The model under review builds one solid part; all positions refer to its coordinate system, in mm. A direction names the side the tool comes from. Round coordinates to 2 decimals unless told otherwise and drop trailing zeros. Loops run counter-clockwise (first coordinate to the right, second up) from the corner with the lowest first, then second, coordinate; pieces in that order, holes last. Notation, with made-up numbers: (29, 67) -> (52, 67) arc R20 cw to (52, 105) -> close; hole circle Ø10 at (62, 47). An arc over 180 degrees is marked (long way). Return JSON: item names as keys, results as strings. Group by question number.
```python
from build123d import *

# Parameters (mm, degrees)
BOSS_EXTRUDE1_DEPTH = 4
CUT_EXTRUDE1_DEPTH  = 5
CUT_EXTRUDE3_DEPTH  = 5
CUT_EXTRUDE4_DEPTH  = 5
CUT_EXTRUDE5_DEPTH  = 5
SHELL1_T            = -1.5


with BuildPart() as part:
    # Sketch1 → Boss-Extrude1 (new body)
    with BuildSketch(Plane(origin=(0, 0, 0), x_dir=(1, 0, 0), z_dir=(0, 1, 0))):
        Polygon((-87.851196474, 52.910261526), (152.148803526, 52.910261526), (182.148803526, 22.910261526), (182.148803526, -167.089738474), (152.148803526, -197.089738474), (-87.851196474, -197.089738474), (-117.851196474, -167.089738474), (-117.851196474, 22.910261526), align=None)
    extrude(amount=BOSS_EXTRUDE1_DEPTH)

    # Sketch2 → Cut-Extrude1 (cut)
    with BuildSketch(Plane(origin=(0, 4, 0), x_dir=(1, 0, 0), z_dir=(0, 1, 0))):
        Polygon((-75.981138789, -72.089738474), (-75.981138789, -32.089738474), (-117.851196474, 9.780319211), (-117.851196474, -153.959796159), (-75.981138789, -112.089738474), align=None)
    extrude(amount=-CUT_EXTRUDE1_DEPTH, mode=Mode.SUBTRACT)

    # Sketch2_5 → Cut-Extrude3 (cut)
    with BuildSketch(Plane(origin=(0, 4, 0), x_dir=(1, 0, 0), z_dir=(0, 1, 0))):
        Polygon((140.278745841, -72.089738474), (140.278745841, -112.089738474), (182.148803526, -153.959796159), (182.148803526, 9.780319211), (140.278745841, -32.089738474), align=None)
    extrude(amount=-CUT_EXTRUDE3_DEPTH, mode=Mode.SUBTRACT)

    # Sketch2_6 → Cut-Extrude4 (cut)
    with BuildSketch(Plane(origin=(0, 4, 0), x_dir=(1, 0, 0), z_dir=(0, 1, 0))):
        Polygon((-61.839003165, 11.040203841), (-90.123274413, 39.324475088), (-104.265410036, 25.182339465), (-75.981138789, -3.101931783), (-68.910070977, 3.969136029), align=None)
        Polygon((126.136610217, 11.040203841), (154.420881465, 39.324475088), (168.563017088, 25.182339465), (140.278745841, -3.101931783), (133.207678029, 3.969136029), align=None)
        Polygon((168.563017088, -169.361816413), (154.420881465, -183.503952036), (126.136610217, -155.219680789), (133.207678029, -148.148612977), (140.278745841, -141.077545165), align=None)
        Polygon((-104.702510795, -169.798917171), (-90.550656516, -183.95077145), (-61.839003165, -155.219680789), (-68.910070977, -148.148612977), (-75.981138789, -141.077545165), align=None)
    extrude(amount=-CUT_EXTRUDE4_DEPTH, mode=Mode.SUBTRACT)

    # Sketch2_7 → Cut-Extrude5 (cut)
    with BuildSketch(Plane(origin=(0, 4, 0), x_dir=(1, 0, 0), z_dir=(0, 1, 0))):
        Polygon((139.018803526, 52.910261526), (32.148803526, 52.910261526), (32.148803526, 11.040203841), (97.148861211, 11.040203841), align=None)
        Polygon((32.148803526, 11.040203841), (32.148803526, 52.910261526), (-74.721196474, 52.910261526), (-32.851138789, 11.040203841), align=None)
        Polygon((-74.721196474, -197.089738474), (32.148803526, -197.089738474), (32.148803526, -155.219680789), (-32.851138789, -155.219680789), align=None)
        Polygon((32.148803526, -155.219680789), (32.148803526, -197.089738474), (139.018803526, -197.089738474), (97.148861211, -155.219680789), align=None)
    extrude(amount=-CUT_EXTRUDE5_DEPTH, mode=Mode.SUBTRACT)

    # Shell1
    shell1_openings = [part.faces().sort_by_distance(p)[0] for p in [
        (147.349813653, 4, 162.290748601),
    ]]
    offset(amount=SHELL1_T, openings=shell1_openings, kind=Kind.INTERSECTION)


solid = part.part
```
1. Wall thickness on line 1 (Z direction, x = -0.5, y = 2.65); line 2 (X direction, y = 0.9, z = -13.5); line 3 (X direction, y = 3.5, z = -2): over which ranges is each line inside the solid? List them lowest first.
2. We need section D-D, the plane x = 18.5. Write out the cut boundary in (y, z).
3. For P1, Ø2, axis at y = 1, z = 80.5, coming from the +X side; P2, Ø1, axis at y = 2.5, z = 115.5, coming from the -X side; P3, Ø1.5, axis at x = -59, z = 141.5, coming from the +Y side, all flat-tipped, find the tip position at first contact; note any pin that passes through.
4. Tool access review of faces 1 (the face through (133.109, 2.028, -4.068)), 2 (the face through (154, 4, -10)), 3 (the face through (-95.12, 2.77, 10.83)): name each direction out of +Z, -Z, +X, -X, +Y, -Y from which nothing blocks a thin tool from reaching the whole face with its end or side.
5. We need section B-B, the plane z = 49. Write out the cut boundary in (x, y), then the cut area to 3 significant figures.
6. We need section C-C, the plane y = 3.05. Give the number of separate pieces and of enclosed holes in the cut face, then the cut area to 3 significant figures.
7. We need section A-A, the plane x = -68. Write out the cut boundary in (y, z).
8. Draft analysis for pull direction X (two halves, no side actions). For faces 4 (the face through (-75.8, 2, -25)), 5 (the face through (-97.21, 2.03, 133.32)), 6 (the face through (34, 0, 70)), state which applies: pulls with the +X half, pulls with the -X half, needs draft (parallel to the pull), parting line crosses it, or undercut.
Check sheet entries:
{
 "1": {"line 1": "z = -11.04 to -9.54, 153.72 to 155.22", "line 2": "x = -117.85 to -92.58, -64.3 to -35.31, 99.61 to 128.6, 156.88 to 182.15", "line 3": "x = -110.07 to -107.95, -83.2 to -81.08, -70.88 to -68.76, 133.06 to 135.18, 145.38 to 147.5, 172.25 to 174.37"},
 "2": {"outline": "(0, -11.04) -> (4, -11.04) -> (4, -9.54) -> (1.5, -9.54) -> (1.5, 153.72) -> (4, 153.72) -> (4, 155.22) -> (0, 155.22) -> close"},
 "3": {"P1": "stops at x = 140.28", "P2": "stops at x = -79.89", "P3": "stops at y = 1.5"},
 "4": {"face 1": "+Y, -Y", "face 2": "+Z, -Z, +X, -X, +Y", "face 3": "+Y"},
 "5": {"outline": "(-75.98, 0) -> (140.28, 0) -> (140.28, 4) -> (138.78, 4) -> (138.78, 1.5) -> (-74.48, 1.5) -> (-74.48, 4) -> (-75.98, 4) -> close", "area": "332 mm²"},
 "6": {"separate pieces": "5", "enclosed holes": "5", "area": "2,500 mm²"},
 "7": {"outline": "(0, -46.19) -> (4, -46.19) -> (4, -44.07) -> (1.5, -44.07) -> (1.5, -19.32) -> (4, -19.32) -> (4, -17.2) -> (0, -17.2) -> close; (0, -4.88) -> (4, -4.88) -> (4, -2.76) -> (1.5, -2.76) -> (1.5, 146.94) -> (4, 146.94) -> (4, 149.06) -> (0, 149.06) -> close; (0, 161.38) -> (4, 161.38) -> (4, 163.51) -> (1.5, 163.51) -> (1.5, 188.25) -> (4, 188.25) -> (4, 190.37) -> (0, 190.37) -> close"},
 "8": {"face 4": "undercut", "face 5": "pulls with the -X half", "face 6": "needs draft"}
}
